Here's how the part is built. I have some questions about the finished solid (model axes, mm). Round coordinates to 2 decimals unless told otherwise and drop trailing zeros. Write each loop counter-clockwise with the first axis right and the second up, starting at its lowest first coordinate (ties: lowest second). Pieces come first, ordered by that corner, then holes. Notation, with made-up numbers: (31.5, -33) -> (53.5, -33) arc R19 ccw to (53.5, -27) -> close; hole circle Ø7 at (-8, 23.25). An arc over 180 degrees is marked (long way). Put each result on its own line as item: value. Start each with the question number.
1) Will this pin go through, and if not, where does the flat tip stop? P1, Ø11.5, axis at x = -431.8, y = 0, coming from the -Z side.
2) I want a section at A-A, the plane y = 0. List the corners of the cut face in (x, z) for me.
3) If I drill on line 1 along Z through (x, y) = (228.6, 8); line 2 along Y through (x, z) = (419.1, -25.5); line 3 along X through (y, z) = (-3.5, 38.5), over which ranges is the centre line in solid material (lowest first)? Write a range as [from, to].
from build123d import *

# Parameters (mm, degrees)
F0_W        = 1066.8
F0_H        = 88.9
F1_DEPTH    = 19.05
F3_W        = 381
F3_H        = 88.9
F4_DEPTH    = 19.05
F10_D       = 12.7
F10_DEPTH   = 609.6
F11_D       = 12.7
F11_DEPTH   = 609.6
F13_D       = 12.7
F13_DEPTH   = 609.6
F13_2_D     = 12.7
F13_2_DEPTH = 609.6
F16_D       = 12.7
F16_DEPTH   = 609.6
F18_D       = 12.7
F18_DEPTH   = 609.6


with BuildPart() as f1:
    # F0 (on Front) → F1 (new body, symmetric)
    with BuildSketch(Plane.XZ):
        Rectangle(F0_W, F0_H)
    extrude(amount=F1_DEPTH, both=True)

    # F3 (on Front) → F4 (join, symmetric)
    with BuildSketch(Plane.XZ):
        Rectangle(F3_W, F3_H)
    extrude(amount=F4_DEPTH, both=True)

    # F11
    with Locations(Plane.XY.offset(152.4)):
        with Locations((419.1, 0)):
            Hole(F11_D / 2, depth=F11_DEPTH)

    # F13
    with Locations(Plane.XZ.offset(91.44)):
        with Locations((-279.4, 0)):
            Hole(F13_D / 2, depth=F13_DEPTH)

    # F16
    with Locations(Plane.XY.offset(152.4)):
        with Locations((-431.8, 0)):
            Hole(F16_D / 2, depth=F16_DEPTH)

    # F18
    with Locations(Plane.XZ.offset(19.05)):
        with Locations((228.6, 0)):
            Hole(F18_D / 2, depth=F18_DEPTH)


with BuildPart() as f2_1:
    # F2: copy of F1
    add(f1.part.moved(Location((0, 114.3, 0))))


with BuildPart() as f6_1:
    # F6: copy of F1
    add(f1.part.moved(Location((0, 152.4, 0))))

    # F10
    with Locations(Plane.XY.offset(152.4)):
        with Locations((419.1, 152.4)):
            Hole(F10_D / 2, depth=F10_DEPTH)

    # F13#2
    with Locations(Plane.XZ.offset(91.44)):
        with Locations((-279.4, 0)):
            Hole(F13_2_D / 2, depth=F13_2_DEPTH)


solid = f1.part
Findings:
1. P1: passes through
2. outline: (-533.4, -44.45) -> (-438.15, -44.45) -> (-438.15, 44.45) -> (-533.4, 44.45) -> close; (-425.45, -44.45) -> (412.75, -44.45) -> (412.75, 44.45) -> (-425.45, 44.45) -> close; (425.45, -44.45) -> (533.4, -44.45) -> (533.4, 44.45) -> (425.45, 44.45) -> close; hole circle Ø12.7 at (-279.4, 0); hole circle Ø12.7 at (228.6, 0)
3. line 1: z = [-44.45, -6.35], [6.35, 44.45]
3. line 2: y = [-19.05, -6.35], [6.35, 19.05]
3. line 3: x = [-533.4, -437.1], [-426.5, 413.8], [424.4, 533.4]
